```python
from build123d import *

# Parameters (mm, degrees)
BOSS_EXTRUDE2_DEPTH = 8.55
SKETCH2_W           = 12
SKETCH2_H           = 3.872399236
CUT_EXTRUDE1_DEPTH  = 10


with BuildPart() as part:
    # Sketch1 → Boss-Extrude2 (new body)
    with BuildSketch(Plane(origin=(0, 0, 0), x_dir=(1, 0, 0), z_dir=(0, 1, 0))):
        with BuildLine():
            Line((0, 3.2), (0, 6.2))
            ThreePointArc((0, 6.2), (0.009618254, 6.199992539), (0.019236485, 6.199970158))
            Line((0.019236485, 6.199970158), (-14.46008445, 23.455752899))
            Line((-14.46008445, 23.455752899), (-20.588439995, 18.313452022))
            Line((-20.588439995, 18.313452022), (-6.10911906, 1.05766928))
            ThreePointArc((-6.10911906, 1.05766928), (-4.749475547, -3.98528318), (-0.019236485, -6.199970158))
            Line((-0.019236485, -6.199970158), (14.46008445, -23.455752899))
            Line((14.46008445, -23.455752899), (20.588439995, -18.313452022))
            Line((20.588439995, -18.313452022), (6.10911906, -1.05766928))
            ThreePointArc((6.10911906, -1.05766928), (6.107470914, -1.067145275), (6.105808069, -1.076618702))
            Line((6.105808069, -1.076618702), (3.15138481, -0.555674169))
            ThreePointArc((3.15138481, -0.555674169), (-2.451342218, -2.056920351), (0, 3.2))
        make_face()
    extrude(amount=BOSS_EXTRUDE2_DEPTH)

    # Sketch2 → Cut-Extrude1 (cut)
    with BuildSketch(Plane(origin=(-3.064177772, 0, 2.571150439), x_dir=(0.64278761, 0, 0.766044443), z_dir=(-0.766044443, 0, 0.64278761))):
        with Locations((-16, 1.936199618)):
            Rectangle(SKETCH2_W, SKETCH2_H)
        with Locations((16, 1.936199618)):
            Rectangle(SKETCH2_W, SKETCH2_H)
    extrude(amount=-CUT_EXTRUDE1_DEPTH, mode=Mode.SUBTRACT)


solid = part.part
```
Part model, mm, in its own coordinate system. A direction names the side the tool comes from. Coordinates: 2 decimals unless noted, no trailing zeros. Order: outer loops, then holes, each group sorted by start corner. A loop starts at its lowest first (then second) coordinate and runs counter-clockwise, first axis right, second up. Notation, with made-up numbers: (-29, -13) - (-24, -13) arc R3 cw to (-24, -9) - close; hole circle Ø7 at (36.5, 39.5). An arc over 180 degrees is marked (long way). Return JSON: item names as keys, results as strings. Group by question number.
Item 1: Which spindle directions (+Z, -Z, +X, -X, +Y, -Y) get a long thin tool onto all of the face, cutting with end or side? Do faces 4 (the face through (-14.18, 1.91, -16.82)), 5 (the face through (-6.5, 1.9, -7.6)), 6 (the face through (17.48, 4.22, 20.92)). Say none if no direction does.
Item 2: Pull direction X, two halves, no side cores. Call faces 1 (the face through (6.38, 1.91, 7.7)), 2 (the face through (-2.385, 4.215, 2.134)), 3 (the face through (-10, 3.872, -12)): pulls with the +X half, pulls with the -X half, needs draft (parallel to the pull), parting line crosses it, or undercut.
Item 3: Drill centre lines: probe 1 along X at (y, z) = (3.75, 0); probe 2 along Z at (x, y) = (-3.5, 7.75); probe 3 along Z at (x, y) = (1, 3.75). Where is each one in solid material? Low to high. Write a range as from..to.
Item 4: Cut at A-A (y = 1). State how many separate pieces and enclosed holes the cut face has, plus the area to 3 significant figures.
Item 5: Cut at B-B (z = 2). List the corners of the cut face in (x, y), plus the area to 3 significant figures.
Item 6: Cut at D-D (x = -8). List the corners of the cut face in (y, z), plus the area to 3 significant figures.
Item 7: Pin check, flat tips, straight feed: pin 1 (1 mm diameter, centred on y = 1, z = -18.5, fed in from +X); pin 2 (5 mm diameter, centred on x = 0, z = 0, fed in from +Y); pin 3 (3.5 mm diameter, centred on y = 4.5, z = -4.5, fed in from +X); pin 4 (2 mm diameter, centred on y = 6.5, z = -13.5, fed in from -X). Stop position of each tip, or through.
Check values:
{
 "1": {"face 4": "+Z, +X, -Y", "face 5": "-Z, -X, -Y", "face 6": "+Z, +X, +Y, -Y"},
 "2": {"face 1": "pulls with the +X half", "face 2": "undercut", "face 3": "needs draft"},
 "3": {"probe 1": "x = -6.2..-3.2", "probe 2": "z = -10.39..5.12", "probe 3": "z = 3.04..7.41"},
 "4": {"separate pieces": "3", "enclosed holes": "0", "area": "216 mm2"},
 "5": {"outline": "(-5.87, 0) - (-2.5, 0) - (-2.5, 8.55) - (-5.87, 8.55) - close; (2.5, 0) - (6.9, 0) - (6.9, 8.55) - (2.5, 8.55) - close", "area": "66.5 mm2"},
 "6": {"outline": "(0, -6.34) - (3.87, -6.34) - (3.87, -15.76) - (8.55, -15.76) - (8.55, -3.31) - (0, -3.31) - close", "area": "70.0 mm2"},
 "7": {"pin 1": "stops at x = -11.58", "pin 2": "passes through", "pin 3": "stops at x = 0.02", "pin 4": "stops at x = -17.39"}
}
